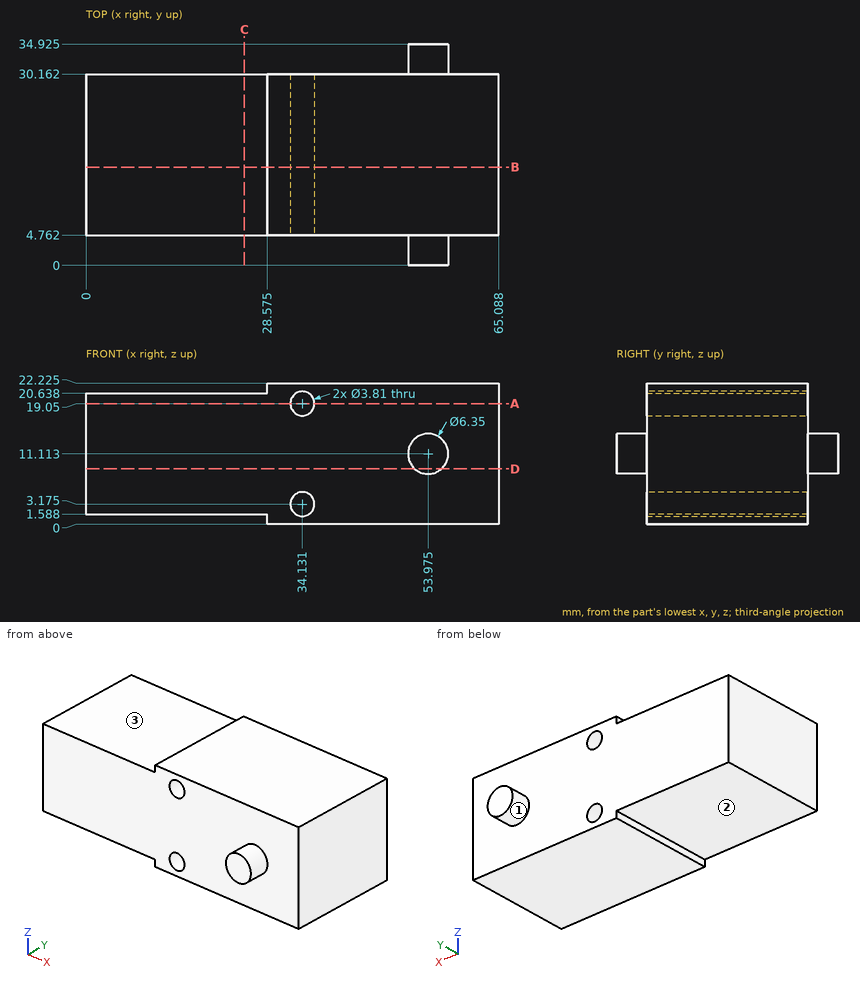
Can you work these out from the drawing? Everything is in mm from the part's minimum corner. A direction names the side the tool comes from. Round coordinates to 2 decimals unless told otherwise and drop trailing zeros. Loops run counter-clockwise (first coordinate to the right, second up) from the corner with the lowest first, then second, coordinate; pieces in that order, holes last. Notation, with made-up numbers: (13, -24.5) -> (38, -24.5) arc R11 cw to (38, -17.5) -> close; hole circle Ø8 at (65.5, 50). An arc over 180 degrees is marked (long way). Put each result on its own line as item: value.
Q1. For pin 1 Ø4 at (x, z) = (21.5, 18.5) entering from +Y; pin 2 Ø2 at (y, z) = (28.5, 3.5) entering from -X; pin 3 Ø6 at (x, z) = (34.13, 19.05) entering from -Y; pin 4 Ø6 at (x, y) = (24, 6.5) entering from +Z, each with a flat end and sliding along its axis, tell me the tip position at first contact or that it passes through.
Checks:
pin 1: y = 30.16
pin 2: x = 0
pin 3: y = 4.76
pin 4: z = 20.64
Q2. I want a section at B-B on y = 15.5. Give the number of separate pieces and of enclosed holes in the cut face, and give its area (3 significant figures).
Checks:
separate pieces: 1
enclosed holes: 2
area: 1,330 mm2
Q3. Which directions (+Z, -Z, +X, -X, +Y, -Y) give clear straight access to the entire face, cutting with the end or side of a thin tool? Please do the marked faces 1, 2 and 3.
Checks:
face 1: +Y
face 2: -Z, -X, +Y, -Y
face 3: +Z, -X, +Y, -Y
Q4. I want a section at C-C on x = 25. Write out the boundary of the cut face in (y, z).
Checks:
outline: (4.76, 1.59) -> (30.16, 1.59) -> (30.16, 20.64) -> (4.76, 20.64) -> close
Q5. I want a section at D-D on z = 8.75. Write out the boundary of the cut face in (x, y) (1 decimal), and give its area (3 significant figures).
Checks:
outline: (0, 4.8) -> (51.9, 4.8) -> (51.9, 0) -> (56.1, 0) -> (56.1, 4.8) -> (65.1, 4.8) -> (65.1, 30.2) -> (56.1, 30.2) -> (56.1, 34.9) -> (51.9, 34.9) -> (51.9, 30.2) -> (0, 30.2) -> close
area: 1,690 mm2
Q6. Please list where these lines run through material, in increasing order: line 1 (X direction, y = 16.25, z = 19.05); line 2 (Z direction, x = 6, y = 24); line 3 (Y direction, x = 43.5, z = 6.5). Write a range as from..to.
Checks:
line 1: 0..32.23, 36.04..65.09
line 2: 1.59..20.64
line 3: 4.76..30.16
Q7. I want a section at A-A on z = 19.05. Write out the boundary of the cut face in (x, y).
Checks:
outline: (0, 4.76) -> (32.23, 4.76) -> (32.23, 30.16) -> (0, 30.16) -> close; (36.04, 4.76) -> (65.09, 4.76) -> (65.09, 30.16) -> (36.04, 30.16) -> close
